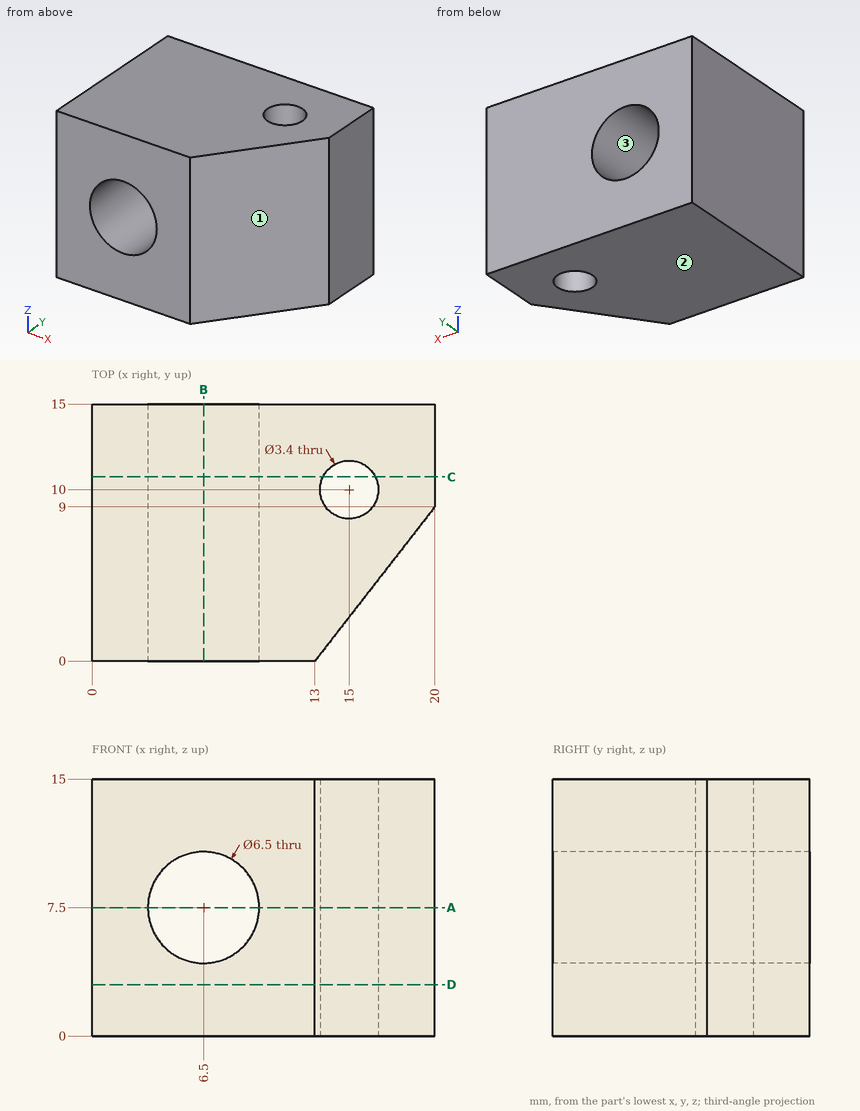
Geometry check sheet. Reference: drawing and pictorial views, mm from the part's lowest x, y, z. Round coordinates to 2 decimals unless told otherwise and drop trailing zeros. Order: outer loops, then holes, each group sorted by start corner. A loop starts at its lowest first (then second) coordinate and runs counter-clockwise, first axis right, second up. Notation, with made-up numbers: M 87,-10.75 L 116,-10.75 A24 cw 116,5.25 Z; hole C 12.5,11 d1. An arc over 180 degrees is marked long. One line per item, written item: value. Start each with the question number.
1. Scan lines: line 1 along Z through (x, y) = (6.5, 7.75); line 2 along X through (y, z) = (11.25, 9.5); line 3 along X through (y, z) = (1.5, 9). Record each from-to range of solid material in increasing order.
2. Section check D-D on z = 3. Enter the section's corners in (x, y), and give its area (3 significant figures).
3. Section check A-A on z = 7.5. Enter the section's corners in (x, y), and give its area (3 significant figures).
4. Section check B-B on x = 6.5. Enter the section's corners in (y, z).
5. Section check C-C on y = 10.75. Enter the section's corners in (x, z).
6. Release check for a two-part mould opening along X. For the marked faces 1, 2 and 3 record: released by +X, released by -X, zero draft, split by the parting line, or undercut.
Results found:
1. line 1: 0 to 4.25, 10.75 to 15
1. line 2: 0 to 3.94, 9.06 to 13.85, 16.15 to 20
1. line 3: 0 to 3.62, 9.38 to 14.17
2. outline: M 0,0 L 13,0 L 20,9 L 20,15 L 0,15 Z; hole C 15,10 d3.4
2. area: 259 mm^2
3. outline: M 0,0 L 3.25,0 L 3.25,15 L 0,15 Z; M 9.75,0 L 13,0 L 20,9 L 20,15 L 9.75,15 Z; hole C 15,10 d3.4
3. area: 162 mm^2
4. outline: M 0,0 L 15,0 L 15,4.25 L 0,4.25 Z; M 0,10.75 L 15,10.75 L 15,15 L 0,15 Z
5. outline: M 0,0 L 13.47,0 L 13.47,15 L 0,15 Z; M 16.53,0 L 20,0 L 20,15 L 16.53,15 Z; hole C 6.5,7.5 d6.5
6. face 1: released by +X
6. face 2: zero draft
6. face 3: undercut
